Part model, mm, in its own coordinate system. A direction names the side the tool comes from. Give positions to 0.01 mm unless a question says otherwise; leave off trailing zeros. Write each loop counter-clockwise with the first axis right and the second up, starting at its lowest first coordinate (ties: lowest second). Pieces come first, ordered by that corner, then holes. Notation, with made-up numbers: (50, 49) - (80, 49) arc R31 ccw to (80, 76) - close; hole circle Ø1 at (-17.75, 39.25). An arc over 180 degrees is marked (long way). Answer in a Markdown table with one row per item. Add a question column.
1. Probe line 1 along Z through (x, y) = (-0.5, 3.7); line 2 along Z through (x, y) = (-0.75, 2.7); line 3 along Z through (x, y) = (-1.5, 0.95). List the from-to ranges inside material, lowest first.
2. Which spindle directions (+Z, -Z, +X, -X, +Y, -Y) get a long thin tool onto all of the face, cutting with end or side? Do faces 1 (the flat face through (0.1, 2.5, 23.5)), 2 (the cylindrical face through (0, 0.5, 16.3)), 3 (the cylindrical face through (-0.1, 2.5, 7.6)), 4 (the cylindrical face through (0, 2, 24)), 5 (the flat face through (-4.3, 0, 22.1)). Say none if no direction does.
3. Band-saw the part on C-C on x = -3.5. Write the cut outline in (y, z).
4. Drop flat-ended pins along their axis: pin 1 Ø1 at (x, y) = (-0.5, 1) entering from -Z; pin 2 Ø6 at (x, z) = (-2.5, 32.5) entering from -Y; pin 3 Ø3 at (x, z) = (3.5, 34.5) entering from +Y; pin 4 Ø1.5 at (y, z) = (4.5, 19.5) entering from +X. Give the stop position or say it passes through.
5. Band-saw the part on B-B on z = 16. Write the cut outline in (x, y).
6. Band-saw the part on D-D on z = 33.5. Write the cut outline in (x, y), plus the area to 3 significant figures.
7. Band-saw the part on A-A on x = 0. Write the cut outline in (y, z).
8. Pull direction Z, two halves, no side cores. Call faces 6 (the cylindrical face through (0, 3, 51)), 7 (the flat face through (0, 3, 0)), 8 (the flat face through (0, 2, 17.5)): released by +Z, released by -Z, zero draft, split by the parting line, or undercut.
```python
from build123d import *

# Parameters (mm, degrees)
F1_ANGLE = 180


with BuildPart() as f1:
    # F0 (on Front) → F1 (revolve)
    with BuildSketch(Plane.XZ):
        Polygon((-4, 50.5), (-3, 50.5), (-3, 51.5), (-5, 51.5), (-5, 0), (-2.5, 0), (-2.5, 15), (-0.5, 15), (-0.5, 17.5), (-4, 17.5), (-4, 23.5), (-2, 23.5), (-2, 24.5), (-4, 24.5), align=None)
    revolve(axis=Axis((0, 0, 15), (0, 0, -1)), revolution_arc=F1_ANGLE)


solid = f1.part
```
Values:
| question | item | result |
|---|---|---|
| 1 | line 1 | z = 0 to 17.5, 23.5 to 24.5, 50.5 to 51.5 |
| 1 | line 2 | z = 0 to 17.5, 23.5 to 24.5 |
| 1 | line 3 | z = 15 to 17.5 |
| 2 | face 1 | -Y |
| 2 | face 2 | +Z, -Z, -Y |
| 2 | face 3 | -Z, -Y |
| 2 | face 4 | +Z, -Y |
| 2 | face 5 | +Z, -Z, +X, -X, -Y |
| 3 | outline | (0, 0) - (3.57, 0) - (3.57, 51.5) - (0, 51.5) - (0, 50.5) - (1.94, 50.5) - (1.94, 24.5) - (0, 24.5) - (0, 23.5) - (1.94, 23.5) - (1.94, 17.5) - (0, 17.5) - close |
| 4 | pin 1 | stops at z = 15 |
| 4 | pin 2 | stops at y = 0 |
| 4 | pin 3 | stops at y = 4.58 |
| 4 | pin 4 | stops at x = 3.31 |
| 5 | outline | (-5, 0) - (-0.5, 0) arc R0.5 cw to (0.5, 0) - (5, 0) arc R5 ccw to start |
| 6 | outline | (-5, 0) - (-4, 0) arc R4 cw to (4, 0) - (5, 0) arc R5 ccw to start |
| 6 | area | 14.1 mm² |
| 7 | outline | (0.5, 15) - (2.5, 15) - (2.5, 0) - (5, 0) - (5, 51.5) - (3, 51.5) - (3, 50.5) - (4, 50.5) - (4, 24.5) - (2, 24.5) - (2, 23.5) - (4, 23.5) - (4, 17.5) - (0.5, 17.5) - close |
| 8 | face 6 | zero draft |
| 8 | face 7 | released by -Z |
| 8 | face 8 | undercut |
